```python
from build123d import *

# Parameters (mm, degrees)
SKETCH1_R           = 57.5
SKETCH1_R_2         = 1.5
BOSS_EXTRUDE1_DEPTH = 5.5
SKETCH3_R           = 2
CUT_EXTRUDE1_DEPTH  = 5.5
SKETCH4_R           = 3.75
CUT_EXTRUDE3_DEPTH  = 5.5
SKETCH5_R           = 3.25
CUT_EXTRUDE4_DEPTH  = 10
SKETCH6_R           = 4
SKETCH6_R_2         = 1.5
CUT_EXTRUDE5_DEPTH  = 10


with BuildPart() as part:
    # Sketch1 → Boss-Extrude1 (new body)
    with BuildSketch(Plane(origin=(0, 0, 0), x_dir=(1, 0, 0), z_dir=(0, 1, 0))):
        Circle(SKETCH1_R)
        with Locations((-52.5, 0)):
            Circle(SKETCH1_R_2, mode=Mode.SUBTRACT)
        with Locations((-26.25, 45.466333699)):
            Circle(SKETCH1_R_2, mode=Mode.SUBTRACT)
        with Locations((26.25, 45.466333699)):
            Circle(SKETCH1_R_2, mode=Mode.SUBTRACT)
        with Locations((52.5, 0)):
            Circle(SKETCH1_R_2, mode=Mode.SUBTRACT)
        with Locations((26.25, -45.466333699)):
            Circle(SKETCH1_R_2, mode=Mode.SUBTRACT)
        with Locations((-26.25, -45.466333699)):
            Circle(SKETCH1_R_2, mode=Mode.SUBTRACT)
    extrude(amount=BOSS_EXTRUDE1_DEPTH)

    # Sketch3 → Cut-Extrude1 (cut)
    with BuildSketch(Plane(origin=(0, 5.5, 0), x_dir=(1, 0, 0), z_dir=(0, 1, 0))):
        with Locations((0, 25.4)):
            Circle(SKETCH3_R)
        with Locations((25.4, 0)):
            Circle(SKETCH3_R)
        with Locations((0, -25.4)):
            Circle(SKETCH3_R)
        with Locations((-25.4, 0)):
            Circle(SKETCH3_R)
    extrude(amount=-CUT_EXTRUDE1_DEPTH, mode=Mode.SUBTRACT)

    # Sketch4 → Cut-Extrude3 (cut)
    with BuildSketch(Plane(origin=(0, 5.5, 0), x_dir=(1, 0, 0), z_dir=(0, 1, 0))):
        with Locations((-30.641777725, 25.711504387)):
            Circle(SKETCH4_R)
        with Locations((25.711504387, 30.641777725)):
            Circle(SKETCH4_R)
        with Locations((30.641777725, -25.711504387)):
            Circle(SKETCH4_R)
        with Locations((-25.711504387, -30.641777725)):
            Circle(SKETCH4_R)
    extrude(amount=-CUT_EXTRUDE3_DEPTH, mode=Mode.SUBTRACT)

    # Sketch5 → Cut-Extrude4 (cut)
    with BuildSketch(Plane.XZ):
        with Locations((-34.641016151, 20)):
            Circle(SKETCH5_R)
    extrude(amount=-CUT_EXTRUDE4_DEPTH, mode=Mode.SUBTRACT)

    # Sketch6 → Cut-Extrude5 (cut)
    with BuildSketch(Plane.XZ):
        with Locations((-10.352761804, -38.637033052)):
            Circle(SKETCH6_R)
        with Locations((32.04293994, -18.5)):
            Circle(SKETCH6_R_2)
        with Locations((26.846787517, -15.5)):
            Circle(SKETCH6_R_2)
    extrude(amount=-CUT_EXTRUDE5_DEPTH, mode=Mode.SUBTRACT)


solid = part.part
```
For this review, take the finished solid that the model builds, in its own axes (mm). Give positions to 0.01 mm unless a question says otherwise; leave off trailing zeros. Loops run counter-clockwise (first coordinate to the right, second up) from the corner with the lowest first, then second, coordinate; pieces in that order, holes last. Notation, with made-up numbers: M 54.5,15 L 107.5,15 A23 cw 107.5,36 Z; hole C 30.25,84.5 d10. An arc over 180 degrees is marked long. One line per item, written item: value. Start each with the question number.
Q1. Add section D-D (x = -16). Give the boundary of the cut face in (y, z).
Q2. Add section A-A (z = 32). Give the boundary of the cut face in (x, y).
Q3. Clearance check with flat-ended pins moving along their axes: pin 1 Ø1 at (x, y) = (16.5, 4) entering from -Z; pin 2 Ø1 at (y, z) = (1.5, 5.5) entering from -X; pin 3 Ø1.5 at (x, y) = (-8, 4.5) entering from +Z. State where each tip first meets the part, or that it passes through.
Q4. Add section B-B (x = 52.5). Give the boundary of the cut face in (y, z), and give its area (3 significant figures).
Q5. Add section C-C (y = 2.65). Count the separate pieces of the cut face and the enclosed holes in it, and give its area (3 significant figures).
Q6. Draft analysis for pull direction Z (two halves, no side actions). For faces 1 (the face through (-1, 5.5, -1)), 2 (the face through (24.75, 2.71, -45.53)), 3 (the face through (25.06, 2.71, 46.38)), state which applies: released by +Z, released by -Z, zero draft, split by the parting line, or undercut.
Q7. For L1, parallel to Z at x = 0, y = 3.35; L2, parallel to X at y = 1.75, z = 0; L3, parallel to X at y = 1.75, z = 28, list the stretches that pass through material, from the lowest coordinate up.
Reply:
1. outline: M 0,-55.23 L 5.5,-55.23 L 5.5,55.23 L 0,55.23 Z
2. outline: M -47.77,0 L -29.21,0 L -29.21,5.5 L -47.77,5.5 Z; M -22.22,0 L 47.77,0 L 47.77,5.5 L -22.22,5.5 Z
3. pin 1: z = -55.23
3. pin 2: x = -57.28
3. pin 3: z = 57.04
4. outline: M 0,-23.45 L 5.5,-23.45 L 5.5,-1.5 L 0,-1.5 Z; M 0,1.5 L 5.5,1.5 L 5.5,23.45 L 0,23.45 Z
4. area: 241 mm²
5. separate pieces: 1
5. enclosed holes: 18
5. area: 10,000 mm²
6. face 1: zero draft
6. face 2: undercut
6. face 3: undercut
7. L1: -57.5 to -27.4, -23.4 to 23.4, 27.4 to 57.5
7. L2: -57.5 to -54, -51 to -27.4, -23.4 to 23.4, 27.4 to 51, 54 to 57.5
7. L3: -50.22 to -28.37, -23.05 to 27.67, 33.61 to 50.22
